The model under review builds one solid part; all positions refer to its coordinate system, in mm. Face numbers are marked on the shaded views. A direction names the side the tool comes from. Give positions to 0.01 mm unless a question says otherwise; leave off trailing zeros. Loops run counter-clockwise (first coordinate to the right, second up) from the corner with the lowest first, then second, coordinate; pieces in that order, holes last. Notation, with made-up numbers: M 30,40.25 L 35,40.25 A28 ccw 35,74.25 Z; hole C 89.5,26.5 d9. An arc over 180 degrees is marked long. Put each result on its own line as item: value. Start each with the question number.
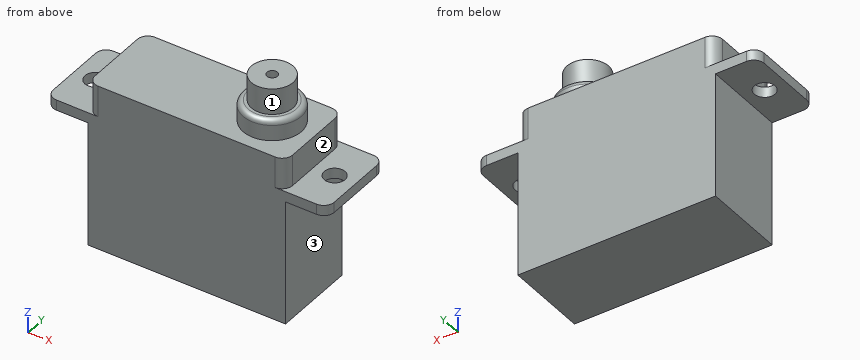
from build123d import *

# Parameters (mm, degrees)
IZIM1_W                     = 19
IZIM1_H                     = 8
Y_KSEKLIK_EKSTR_ZYON1_DEPTH = 12
IZIM2_R                     = 1
Y_KSEKLIK_EKSTR_ZYON2_DEPTH = 1
Y_KSEKLIK_EKSTR_ZYON3_DEPTH = 3
IZIM4_R                     = 2.8
Y_KSEKLIK_EKSTR_ZYON4_DEPTH = 2
IZIM5_R                     = 2
Y_KSEKLIK_EKSTR_ZYON5_DEPTH = 2.5
IZIM6_R                     = 0.5
KES_EKSTR_ZYON1_DEPTH       = 5
RADYUS1_R                   = 0.5


with BuildPart() as part:
    # Çizim1 → Yükseklik-Ekstrüzyon1 (new body)
    with BuildSketch(Plane.XY):
        Rectangle(IZIM1_W, IZIM1_H)
    extrude(amount=Y_KSEKLIK_EKSTR_ZYON1_DEPTH)

    # Çizim2 → Yükseklik-Ekstrüzyon2 (add)
    with BuildSketch(Plane.XY.offset(12)):
        with BuildLine():
            Line((-12.5, -4), (12.5, -4))
            ThreePointArc((12.5, -4), (13.207106781, -3.707106781), (13.5, -3))
            Line((13.5, -3), (13.5, 3))
            ThreePointArc((13.5, 3), (13.207106781, 3.707106781), (12.5, 4))
            Line((12.5, 4), (-12.5, 4))
            ThreePointArc((-12.5, 4), (-13.207106781, 3.707106781), (-13.5, 3))
            Line((-13.5, 3), (-13.5, -3))
            ThreePointArc((-13.5, -3), (-13.207106781, -3.707106781), (-12.5, -4))
        make_face()
        with Locations((-11.5, 0)):
            Circle(IZIM2_R, mode=Mode.SUBTRACT)
        with Locations((11.5, 0)):
            Circle(IZIM2_R, mode=Mode.SUBTRACT)
    extrude(amount=Y_KSEKLIK_EKSTR_ZYON2_DEPTH)

    # Çizim3 → Yükseklik-Ekstrüzyon3 (add)
    with BuildSketch(Plane.XY.offset(13)):
        with BuildLine():
            Line((-8.5, -4), (8.5, -4))
            ThreePointArc((8.5, -4), (9.207106781, -3.707106781), (9.5, -3))
            Line((9.5, -3), (9.5, 3))
            ThreePointArc((9.5, 3), (9.207106781, 3.707106781), (8.5, 4))
            Line((8.5, 4), (-8.5, 4))
            ThreePointArc((-8.5, 4), (-9.207106781, 3.707106781), (-9.5, 3))
            Line((-9.5, 3), (-9.5, -3))
            ThreePointArc((-9.5, -3), (-9.207106781, -3.707106781), (-8.5, -4))
        make_face()
    extrude(amount=Y_KSEKLIK_EKSTR_ZYON3_DEPTH)

    # Çizim4 → Yükseklik-Ekstrüzyon4 (add)
    with BuildSketch(Plane.XY.offset(16)):
        with Locations((5.5, 0)):
            Circle(IZIM4_R)
    extrude(amount=Y_KSEKLIK_EKSTR_ZYON4_DEPTH)

    # Çizim5 → Yükseklik-Ekstrüzyon5 (add)
    with BuildSketch(Plane.XY.offset(18)):
        with Locations((5.5, 0)):
            Circle(IZIM5_R)
    extrude(amount=Y_KSEKLIK_EKSTR_ZYON5_DEPTH)

    # Çizim6 → Kes-Ekstrüzyon1 (cut)
    with BuildSketch(Plane.XY.offset(20.5)):
        with Locations((5.5, 0)):
            Circle(IZIM6_R)
    extrude(amount=-KES_EKSTR_ZYON1_DEPTH, mode=Mode.SUBTRACT)

    # Radyus1
    radyus1_edges = [part.edges().sort_by_distance(p)[0] for p in [
        (2.7, 0, 18),
    ]]
    fillet(radyus1_edges, radius=RADYUS1_R)


solid = part.part
(1) We need section D-D, the plane z = 19.25. Write out the cut boundary in (x, y), plus the area to 3 significant figures.
(2) For the marked faces 1, 2 and 3, list the 3-axis set-ups (+Z, -Z, +X, -X, +Y, -Y) from which the entire face can be reached by the end or side of a thin tool; tool diameter is ignored.
(3) Insertion check: pin 1 (3 mm diameter, centred on x = -11.5, y = -0.5, fed in from -Z); pin 2 (0.9 mm diameter, centred on y = 0, z = 14.5, fed in from +X); pin 3 (4 mm diameter, centred on y = -2, z = 3, fed in from -X). Each pin has a flat end and moves straight along its axis. Give the tip position at first contact, or say it passes through.
(4) We need section A-A, the plane x = -11.5. Write out the cut boundary in (y, z).
(5) We need section B-B, the plane y = 0. State how many separate pieces and enclosed holes the cut face has, plus the area to 3 significant figures.
(6) To check wall thickness, follow L1, parallel to Y at x = -11.5, z = 12.8; L2, parallel to Y at x = 5.5, z = 17.5; L3, parallel to X at y = -2.25, z = 11.5. State the ranges of each line that lie inside material, in increasing order. Write a range as [from, to].
(7) We need section C-C, the plane x = 5.5. Write out the cut boundary in (y, z), plus the area to 3 significant figures.
Check sheet entries:
1. outline: C 5.5,0 d4; hole C 5.5,0 d1
1. area: 11.8 mm²
2. face 1: +Z
2. face 2: +Z, +X, +Y, -Y
2. face 3: -Z, +X, +Y, -Y
3. pin 1: stops at z = 12
3. pin 2: stops at x = 9.5
3. pin 3: stops at x = -9.5
4. outline: M -4,12 L -1,12 L -1,13 L -4,13 Z; M 1,12 L 4,12 L 4,13 L 1,13 Z
5. separate pieces: 3
5. enclosed holes: 0
5. area: 324 mm²
6. L1: y = [-4, -1], [1, 4]
6. L2: y = [-2.8, -0.5], [0.5, 2.8]
6. L3: x = [-9.5, 9.5]
7. outline: M -4,0 L 4,0 L 4,16 L 2.8,16 L 2.8,17.5 A0.5 ccw 2.3,18 L 2,18 L 2,20.5 L 0.5,20.5 L 0.5,15.5 L -0.5,15.5 L -0.5,20.5 L -2,20.5 L -2,18 L -2.3,18 A0.5 ccw -2.8,17.5 L -2.8,16 L -4,16 Z
7. area: 144 mm²
